Part model, mm, in its own coordinate system. Coordinates: 2 decimals unless noted, no trailing zeros. Loops run counter-clockwise (first coordinate to the right, second up) from the corner with the lowest first, then second, coordinate; pieces in that order, holes last. Notation, with made-up numbers: (50, 74.5) -> (105, 74.5) arc R18 ccw to (105, 83.5) -> close; hole circle Ø5 at (17.25, -17.5). An arc over 180 degrees is marked (long way). One line per question, with ' | ' between items. Start each with the question number.
1) Cut at A-A (z = -11.5). List the corners of the cut face in (x, y).
2) Cut at B-B (y = 12.5). List the corners of the cut face in (x, z).
3) Cut at C-C (x = 0). List the corners of the cut face in (y, z), plus the area to 3 significant figures.
4) Cut at D-D (z = -20.5). List the corners of the cut face in (x, y).
5) Probe L1, parallel to X at y = 7.5, z = -5; L2, parallel to X at y = -1, z = -3.5; L3, parallel to Z at x = 5.5, y = -12. List the from-to ranges inside material, lowest first. Write a range as from..to.
6) Two-plate mould, pull along X, no slides. Class faces 1 (the face through (-0.473, -0.21, -21.495)), 2 (the face through (-31, 0, 0)), 3 (the face through (40, 0, -15)): released by +X, released by -X, zero draft, split by the parting line, or undercut.
Solid Edge part; units mm, degrees
sketch "Sketch1" plane through (0, 0, 0) normal (0, 0, 1) x (1, 0, 0)
  line L0 (-40, -15) -> (40, -15)
  line L1 (40, -15) -> (40, 15)
  line L2 (40, 15) -> (-40, 15)
  line L3 (-40, 15) -> (-40, -15)
extrude "Protrusion1" add sketch "Sketch1" against normal blind 30
sketch "Sketch2" plane through (0, -15, -15) normal (0, -1, 0) x (1, 0, 0)
  circle A0 centre (0, 15) radius 21.5
extrude "Recorte_Extrudado_1" cut sketch "Sketch2" against normal blind 30
Reported:
1) outline: (-40, -15) -> (-18.17, -15) -> (-18.17, 15) -> (-40, 15) -> close; (18.17, -15) -> (40, -15) -> (40, 15) -> (18.17, 15) -> close
2) outline: (-40, -30) -> (40, -30) -> (40, 0) -> (21.5, 0) arc R21.5 cw to (-21.5, 0) -> (-40, 0) -> close
3) outline: (-15, -30) -> (15, -30) -> (15, -21.5) -> (-15, -21.5) -> close | area: 255 mm²
4) outline: (-40, -15) -> (-6.48, -15) -> (-6.48, 15) -> (-40, 15) -> close; (6.48, -15) -> (40, -15) -> (40, 15) -> (6.48, 15) -> close
5) L1: x = -40..-20.91, 20.91..40 | L2: x = -40..-21.21, 21.21..40 | L3: z = -30..-20.78
6) face 1: undercut | face 2: zero draft | face 3: released by +X
